Read the model definition and answer for the solid it produces. Units are mm, in the model's axes. A direction names the side the tool comes from. Give positions to 0.01 mm unless a question says otherwise; leave off trailing zeros. Loops run counter-clockwise (first coordinate to the right, second up) from the corner with the lowest first, then second, coordinate; pieces in that order, holes last. Notation, with made-up numbers: (8, -33.75) -> (15, -33.75) arc R20 ccw to (15, -15.75) -> close; hole circle Ø4 at (63, -21). An arc over 180 degrees is marked (long way). One line per item, written item: value. Start each with the question number.
from build123d import *

# Parameters (mm, degrees)
SKETCH_W        = 30
SKETCH_H        = 40
PAD_DEPTH       = 9
SKETCH002_W     = 30
SKETCH002_H     = 5
PAD001_DEPTH    = 30
SKETCH003_R     = 2
SKETCH003_R_2   = 4
POCKET_DEPTH    = 5.001
POCKET001_DEPTH = 2
SKETCH007_W     = 30
SKETCH007_H     = 5
PAD002_DEPTH    = 20
SKETCH008_R     = 4
POCKET002_DEPTH = 9.001
POCKET003_DEPTH = 5


with BuildPart() as part:
    # Sketch → Pad (new body)
    with BuildSketch(Plane.XY):
        with Locations((-10.97123, 13.069184)):
            Rectangle(SKETCH_W, SKETCH_H)
    extrude(amount=PAD_DEPTH)

    # Sketch002 (on Face6 of Pad) → Pad001 (join)
    with BuildSketch(Plane.XY.offset(9)):
        with Locations((-10.97123, 30.569184)):
            Rectangle(SKETCH002_W, SKETCH002_H)
    extrude(amount=PAD001_DEPTH)

    # Sketch003 (on Face11 of Pad001) → Pocket (cut, through all)
    with BuildSketch(Plane.XZ.offset(-28.069184)):
        with Locations((-1.97123, 33)):
            Circle(SKETCH003_R)
        with Locations((-19.97123, 33)):
            Circle(SKETCH003_R)
        with Locations((-19.97123, 15)):
            Circle(SKETCH003_R)
        with Locations((-1.97123, 15)):
            Circle(SKETCH003_R)
        with Locations((-10.97123, 24)):
            Circle(SKETCH003_R_2)
    extrude(amount=-POCKET_DEPTH, mode=Mode.SUBTRACT)

    # Sketch005 (on Face16 of Pocket) → Pocket001 (cut)
    with BuildSketch(Plane.XZ.offset(-28.069184)):
        Polygon((-4.47123, 27.752777), (-10.97123, 31.505553), (-17.47123, 27.752777), (-17.47123, 20.247223), (-10.97123, 16.494447), (-4.47123, 20.247223), align=None)
    extrude(amount=-POCKET001_DEPTH, mode=Mode.SUBTRACT)

    # Sketch007 (on Face7 of Pocket001) → Pad002 (join)
    with BuildSketch(Plane.XY.offset(9)):
        with Locations((-10.97123, -4.430816)):
            Rectangle(SKETCH007_W, SKETCH007_H)
    extrude(amount=PAD002_DEPTH)

    # Sketch008 (on Face8 of Pad002) → Pocket002 (cut, through all)
    with BuildSketch(Plane.XY.offset(9)):
        with Locations((-10.97123, 13.069184)):
            Circle(SKETCH008_R)
    extrude(amount=-POCKET002_DEPTH, mode=Mode.SUBTRACT)

    # Sketch009 (on Face8 of Pocket002) → Pocket003 (cut)
    with BuildSketch(Plane.XY.offset(9)):
        Polygon((-4.47123, 16.821961), (-10.97123, 20.574738), (-17.47123, 16.821961), (-17.47123, 9.316407), (-10.97123, 5.563631), (-4.47123, 9.316407), align=None)
    extrude(amount=-POCKET003_DEPTH, mode=Mode.SUBTRACT)


solid = part.part
Item 1: Determine the mould class of faces 1 (the flat face through (-7.676, 29.055, 29.603)), 2 (the flat face through (-11, 18, 0)), 3 (the flat face through (-18, 28.069, 24)), 4 (the cylindrical face through (-19.048, 30.534, 31.226)) for opening direction Z: pulls with the +Z half, pulls with the -Z half, needs draft (parallel to the pull), parting line crosses it, or undercut.
Item 2: Flat-ended cylindrical pins translate along their axes: pin 1 (12 mm diameter, centred on y = 8.5, z = 26.5, fed in from -X); pin 2 (9 mm diameter, centred on x = -10.97, y = 13.07, fed in from +Z); pin 3 (2 mm diameter, centred on x = -12, z = 23, fed in from +Y); pin 4 (14.5 mm diameter, centred on x = -8.5, y = 13, fed in from +Z). Find the tip coordinate at first contact, or state that the pin passes through.
Item 3: Section D-D, the plane y = 11 is taken. Determine the outline of the cut face in (x, z).
Item 4: For faces 5 (the flat face through (-17.471, 29, 24)), 6 (the flat face through (-14, 10, 4)), 7 (the flat face through (-18, 13, 9)), determine the directions among +Z, -Z, +X, -X, +Y, -Y from which every point of the face is accessible in a straight line to the end or side of a thin tool.
Item 5: Section B-B, the plane z = 5.5 is taken. Determine the outline of the cut face in (x, y), plus the area to 3 significant figures.
Item 6: Consider L1, parallel to Y at x = 0.25, z = 23.5; L2, parallel to Y at x = -7.5, z = 19.5; L3, parallel to Y at x = -10.75, z = 30. Determine where each line is inside the solid, lowest interval first. Write a range as [from, to].
Item 7: Section C-C, the plane x = -12 is taken. Determine the outline of the cut face in (y, z).
Item 8: Section A-A, the plane z = 33 is taken. Determine the outline of the cut face in (x, y), plus the area to 3 significant figures.
Computed values:
1. face 1: undercut
1. face 2: pulls with the -Z half
1. face 3: needs draft
1. face 4: undercut
2. pin 1: through
2. pin 2: z = 4
2. pin 3: y = -1.93
2. pin 4: z = 9
3. outline: (-25.97, 0) -> (-14.39, 0) -> (-14.39, 4) -> (-17.47, 4) -> (-17.47, 9) -> (-25.97, 9) -> close; (-7.55, 0) -> (4.03, 0) -> (4.03, 9) -> (-4.47, 9) -> (-4.47, 4) -> (-7.55, 4) -> close
4. face 5: none
4. face 6: +Z
4. face 7: +Z, +X, -X
5. outline: (-25.97, -6.93) -> (4.03, -6.93) -> (4.03, 33.07) -> (-25.97, 33.07) -> close; hole (-17.47, 9.32) -> (-10.97, 5.56) -> (-4.47, 9.32) -> (-4.47, 16.82) -> (-10.97, 20.57) -> (-17.47, 16.82) -> close
5. area: 1,050 mm²
6. L1: [-6.93, -1.93], [28.07, 33.07]
6. L2: [-6.93, -1.93], [30.07, 33.07]
6. L3: [30.07, 33.07]
7. outline: (-6.93, 0) -> (9.2, 0) -> (9.2, 4) -> (6.16, 4) -> (6.16, 9) -> (-1.93, 9) -> (-1.93, 29) -> (-6.93, 29) -> close; (16.93, 0) -> (33.07, 0) -> (33.07, 20.13) -> (30.07, 20.13) -> (30.07, 17.09) -> (28.07, 17.09) -> (28.07, 9) -> (19.98, 9) -> (19.98, 4) -> (16.93, 4) -> close; (28.07, 30.91) -> (30.07, 30.91) -> (30.07, 27.87) -> (33.07, 27.87) -> (33.07, 39) -> (28.07, 39) -> close
8. outline: (-25.97, 28.07) -> (-21.97, 28.07) -> (-21.97, 33.07) -> (-25.97, 33.07) -> close; (-17.97, 28.07) -> (-3.97, 28.07) -> (-3.97, 33.07) -> (-17.97, 33.07) -> close; (0.03, 28.07) -> (4.03, 28.07) -> (4.03, 33.07) -> (0.03, 33.07) -> close
8. area: 110 mm²
